Design review of the part shown in the three views and the two pictorial views. Dimensions are in mm from the part's minimum x, y and z. Coordinates: 2 decimals unless noted, no trailing zeros. Loops run counter-clockwise (first coordinate to the right, second up) from the corner with the lowest first, then second, coordinate; pieces in that order, holes last.
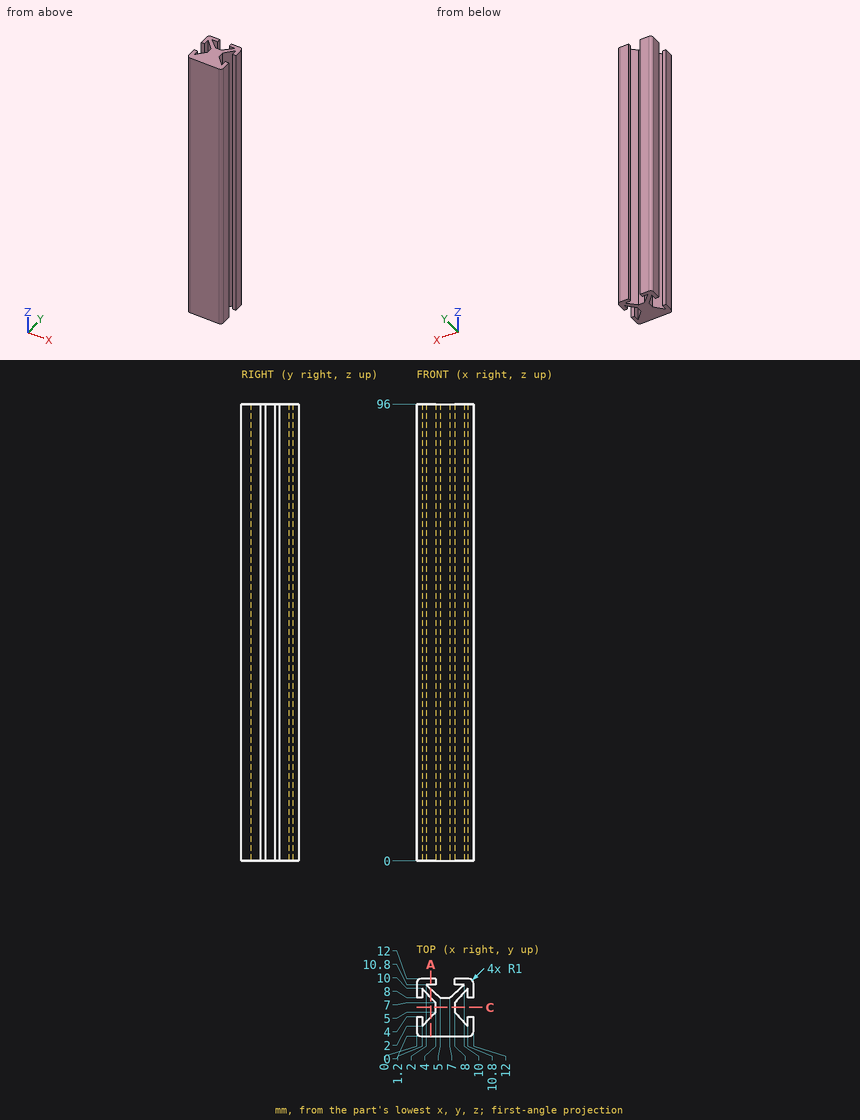
Q1. Wall thickness on probe 1 along Y at (x, z) = (2.5, 54.5); probe 2 along Y at (x, z) = (2.25, 51.5) (3 decimals); probe 3 along X at (y, z) = (8.75, 48): over which ranges is each line inside the solid? List them lowest first.
Q2. For pin 1 Ø0.6 at (x, z) = (11.5, 33.5) entering from -Y; pin 2 Ø1.6 at (y, z) = (6.5, 55.5) entering from -X; pin 3 Ø1.6 at (x, z) = (6, 34.5) entering from +Y, all flat-tipped, find the tip position at first contact; note any pin that passes through.
Q3. Consider section A-A (x = 3). State the section outline as (y, z) points, then the cut area to 3 significant figures.
Q4. Consider section C-C (y = 6). State the section outline as (x, z) points, then the cut area to 3 significant figures.
Model answer:
1. probe 1: y = 0 to 3.39, 8.61 to 10.33, 10.8 to 12
1. probe 2: y = 0 to 3.125, 8.875 to 10.567, 10.8 to 12
1. probe 3: x = 0 to 1.2, 2.37 to 4.2, 7.8 to 9.63, 10.8 to 12
2. pin 1: stops at y = 0.02
2. pin 2: stops at x = 3.72
2. pin 3: stops at y = 8
3. outline: (0, 0) - (3.93, 0) - (3.93, 96) - (0, 96) - close; (8.07, 0) - (9.87, 0) - (9.87, 96) - (8.07, 96) - close; (10.8, 0) - (12, 0) - (12, 96) - (10.8, 96) - close
3. area: 665 mm2
4. outline: (4, 0) - (8, 0) - (8, 96) - (4, 96) - close
4. area: 384 mm2
